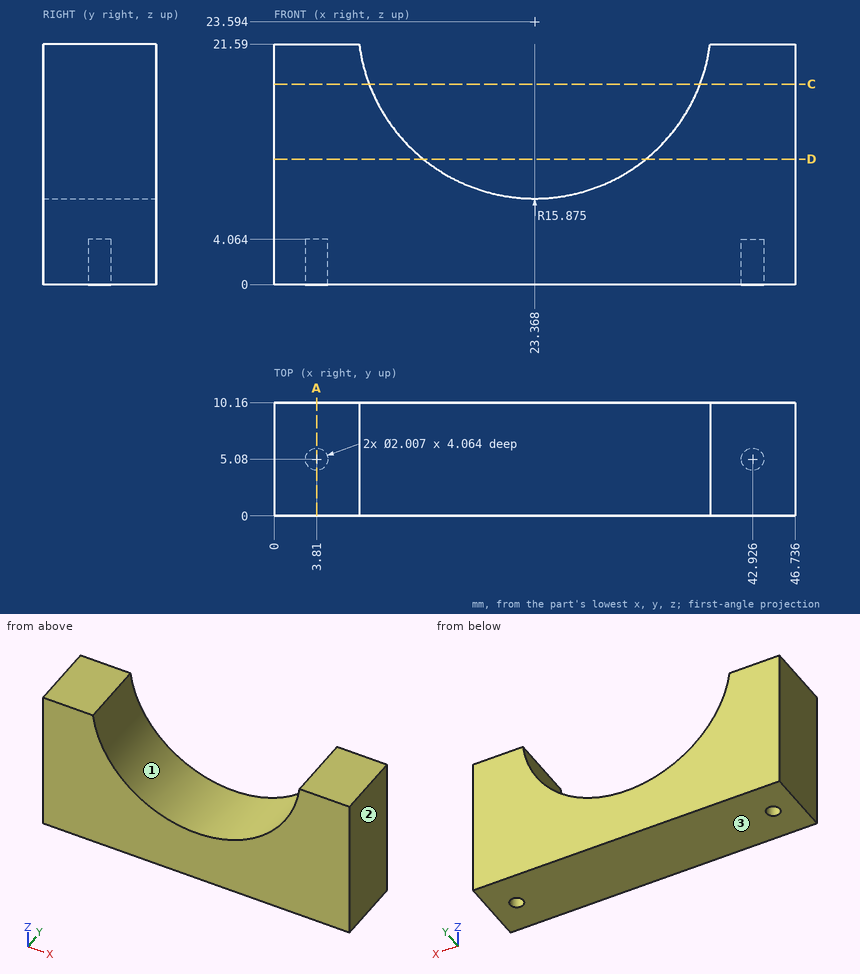
Study the drawing (mm; zero at the part's minimum x, y, z) and answer. Give positions to 0.01 mm unless a question says otherwise; leave off trailing zeros. Loops run counter-clockwise (first coordinate to the right, second up) from the corner with the lowest first, then second, coordinate; pieces in that order, holes last. Notation, with made-up numbers: (-21.75, -5.5) - (-3.75, -5.5) arc R21 cw to (-3.75, 15.5) - close; hole circle Ø3 at (56.25, 85.25). An arc over 180 degrees is marked (long way). Return JSON: item names as keys, results as strings. Group by question number.
1. Straight lines are drawn through the part: line 1 (X direction, y = 5.08, z = 1.55); line 2 (Y direction, x = 3.81, z = 1.65); line 3 (X direction, y = 1.5, z = 16.5) (1 decimal). For each, find the intervals that lie inside material, in ascending order. Write a range as [from, to].
2. Find section A-A (x = 3.81). Write down the section's boundary in (y, z), then the cut area to 3 significant figures.
3. Find section C-C (z = 18). Write down the section's boundary in (x, y) (1 decimal), then the cut area to 3 significant figures.
4. Determine the mould class of the marked faces 1, 2 and 3 for opening direction X: pulls with the +X half, pulls with the -X half, needs draft (parallel to the pull), parting line crosses it, or undercut.
5. Find section D-D (z = 11.25). Write down the section's boundary in (x, y), then the cut area to 3 significant figures.
6. Given pin 1 Ø1.8 at (x, y) = (3.81, 5.08) entering from -Z, flat-ended and moving along its own axis, determine where the tip first touches the part or whether it passes through.
Verdict:
{
 "1": {"line 1": "x = [0, 2.81], [4.81, 41.92], [43.93, 46.74]", "line 2": "y = [0, 4.08], [6.08, 10.16]", "line 3": "x = [0, 9.2], [37.6, 46.7]"},
 "2": {"outline": "(0, 0) - (4.08, 0) - (4.08, 4.06) - (6.08, 4.06) - (6.08, 0) - (10.16, 0) - (10.16, 21.59) - (0, 21.59) - close", "area": "211 mm^2"},
 "3": {"outline": "(0, 0) - (8.5, 0) - (8.5, 10.2) - (0, 10.2) - close; (38.2, 0) - (46.7, 0) - (46.7, 10.2) - (38.2, 10.2) - close", "area": "173 mm^2"},
 "4": {"face 1": "undercut", "face 2": "pulls with the +X half", "face 3": "needs draft"},
 "5": {"outline": "(0, 0) - (13.39, 0) - (13.39, 10.16) - (0, 10.16) - close; (33.35, 0) - (46.74, 0) - (46.74, 10.16) - (33.35, 10.16) - close", "area": "272 mm^2"},
 "6": {"pin 1": "stops at z = 4.06"}
}
